Geometry: final body of the model. Coordinates: model frame, mm. A direction names the side the tool comes from. Give positions to 0.01 mm unless a question says otherwise; leave off trailing zeros. Write each loop counter-clockwise with the first axis right and the second up, starting at its lowest first coordinate (ties: lowest second). Pieces come first, ordered by that corner, then holes.
```python
from build123d import *

# Parameters (mm, degrees)
RESSALTO_EXTRUS_O1_DEPTH = 39.4
ESBO_O2_W                = 3.7
ESBO_O2_H                = 2.5
CORTE_EXTRUS_O1_DEPTH    = 46.281121894
ESBO_O3_W                = 3.7
ESBO_O3_H                = 2
CORTE_EXTRUS_O2_DEPTH    = 10
PADR_O_LINEAR1_COUNT     = 4
PADR_O_LINEAR1_PITCH     = 6.1
ESBO_O5_W                = 1.5
ESBO_O5_H                = 7.6
RESSALTO_EXTRUS_O2_DEPTH = 1


with BuildPart() as part:
    # Esboço1 → Ressalto-extrusão1 (new body)
    with BuildSketch(Plane.XY):
        Polygon((0, 0), (0, 10.1), (3.7, 10.1), (3.7, 2.5), (11.7, 2.5), (11.7, 4), (19.9, 4), (19.9, 0), (3.7, 0), (3.7, -1), (0, -1), align=None)
    extrude(amount=-RESSALTO_EXTRUS_O1_DEPTH)

    # Esboço2 → Corte-extrusão1 (cut, through all)
    with BuildSketch(Plane(origin=(19.9, 0, 0), x_dir=(0, 0, -1), z_dir=(1, 0, 0))):
        with Locations((11.9, 1.25)):
            Rectangle(ESBO_O2_W, ESBO_O2_H)
    corte_extrus_o1 = extrude(amount=-CORTE_EXTRUS_O1_DEPTH, mode=Mode.SUBTRACT)

    # Esboço3 → Corte-extrusão2 (cut)
    with BuildSketch(Plane(origin=(3.7, 0, 0), x_dir=(0, 0, -1), z_dir=(1, 0, 0))):
        with Locations((11.9, 6.914453418)):
            Rectangle(ESBO_O3_W, ESBO_O3_H)
    corte_extrus_o2 = extrude(amount=-CORTE_EXTRUS_O2_DEPTH, mode=Mode.SUBTRACT)

    # Padrão linear1: Corte-extrusão1, Corte-extrusão2 ×4
    with Locations(*[(0, 0, -i * PADR_O_LINEAR1_PITCH) for i in range(1, PADR_O_LINEAR1_COUNT)]):
        add(corte_extrus_o1, mode=Mode.SUBTRACT)
        add(corte_extrus_o2, mode=Mode.SUBTRACT)

    # Esboço5 → Ressalto-extrusão2 (add)
    with BuildSketch(Plane(origin=(3.7, 0, 0), x_dir=(0, 0, -1), z_dir=(1, 0, 0))):
        with Locations((0.75, 6.3)):
            Rectangle(ESBO_O5_W, ESBO_O5_H)
    ressalto_extrus_o2 = extrude(amount=RESSALTO_EXTRUS_O2_DEPTH)

    # Espelhar1: Ressalto-extrusão2 across plane
    add(ressalto_extrus_o2.mirror(Plane.XY.offset(-19.7)))


solid = part.part
```
Item 1: Line query: L1, parallel to Z at x = 4, y = 7; L2, parallel to Y at x = 9.5, z = -7; L3, parallel to X at y = 8.5, z = -18.5. Output: solid intervals per line, ascending.
Found:
L1: z = -39.4 to -37.9, -1.5 to 0
L2: y = 0 to 2.5
L3: x = 0 to 3.7
Item 2: Reachability of faces 1 (the face through (4.7, 6, -1)), 2 (the face through (3.7, -0.5, -19.4)), 3 (the face through (10, 1, -32.05)) from +Z, -Z, +X, -X, +Y, -Y: full face, straight path, thin tool, end or side. Return the list, or none.
Found:
face 1: +Z, -Z, +Y
face 2: +Z, -Z, +X, -Y
face 3: +X, -X
Item 3: Section D-D, the plane y = 5.5. Return the cut outline in (x, z).
Found:
outline: (0, -39.4) - (4.7, -39.4) - (4.7, -37.9) - (3.7, -37.9) - (3.7, -1.5) - (4.7, -1.5) - (4.7, 0) - (0, 0) - close
Item 4: Section A-A, the plane z = -30.5. Return the cut outline in (x, y).
Found:
outline: (0, -1) - (3.7, -1) - (3.7, 0) - (0, 0) - close; (0, 2.5) - (3.7, 2.5) - (3.7, 5.91) - (0, 5.91) - close; (0, 7.91) - (3.7, 7.91) - (3.7, 10.1) - (0, 10.1) - close; (11.7, 2.5) - (19.9, 2.5) - (19.9, 4) - (11.7, 4) - close
Item 5: Pull-direction query (Z, two-part tool) for faces 4 (the face through (11.7, 3, -19)), 5 (the face through (3.7, 5.5, -19.4)); classes: +Z half, -Z half, draft (parallel to the pull), parting line (faces both ways), or undercut.
Found:
face 4: draft
face 5: undercut
Item 6: Section B-B, the plane y = 1.5. Return the cut outline in (x, z), plus the area to 3 significant figures.
Found:
outline: (0, -39.4) - (19.9, -39.4) - (19.9, -32.05) - (0, -32.05) - close; (0, -28.35) - (19.9, -28.35) - (19.9, -25.95) - (0, -25.95) - close; (0, -22.25) - (19.9, -22.25) - (19.9, -19.85) - (0, -19.85) - close; (0, -16.15) - (19.9, -16.15) - (19.9, -13.75) - (0, -13.75) - close; (0, -10.05) - (19.9, -10.05) - (19.9, 0) - (0, 0) - close
area: 490 mm2
Item 7: Section C-C, the plane x = 6.75. Return the cut outline in (y, z).
Found:
outline: (0, -39.4) - (2.5, -39.4) - (2.5, -32.05) - (0, -32.05) - close; (0, -28.35) - (2.5, -28.35) - (2.5, -25.95) - (0, -25.95) - close; (0, -22.25) - (2.5, -22.25) - (2.5, -19.85) - (0, -19.85) - close; (0, -16.15) - (2.5, -16.15) - (2.5, -13.75) - (0, -13.75) - close; (0, -10.05) - (2.5, -10.05) - (2.5, 0) - (0, 0) - close
Item 8: Pin query (flat end, axial travel): pin 1 Ø2.5 at (x, z) = (9.5, -20.5) entering from +Y; pin 2 Ø10 at (x, z) = (9.5, -14.5) entering from +Y; pin 3 Ø1.1 at (x, z) = (16, -17.5) entering from -Y. Return the tip coordinate at first contact, or that it passes through.
Found:
pin 1: stops at y = 2.5
pin 2: stops at y = 4
pin 3: stops at y = 2.5
